Check sheet for the modelled part. Datum: model origin and axes. Units: mm. A direction names the side the tool comes from. Round coordinates to 2 decimals unless told otherwise and drop trailing zeros. Order: outer loops, then holes, each group sorted by start corner. A loop starts at its lowest first (then second) coordinate and runs counter-clockwise, first axis right, second up.
Q1. Depth check by flat-ended pin: P1, Ø12.5, axis at y = 3.5, z = 27, coming from the -X side; P2, Ø8, axis at x = 6, z = 4.5, coming from the +Y side; P3, Ø10, axis at y = 14.5, z = 23, coming from the -X side; P4, Ø5.5, axis at y = -0.5, z = 9.5, coming from the +X side. Enter the tip coordinate at first touch or a pass-through.
Q2. Cross-section at C-C on y = 0. Give the number of separate pieces and of enclosed holes in the cut face, then the cut area to 3 significant figures.
Q3. Cross-section at A-A on y = -16. Record the cut outline in (x, z), then the cut area to 3 significant figures.
Q4. Set-up check for faces 4 (the flat face through (1.5, 0, 27)), 5 (the flat face through (-9, 0, 11)), 6 (the cylindrical face through (-8.4, -6.93, 10.92)), 7 (the cylindrical face through (-3, 0, 28)), 8 (the flat face through (3, -4, 27)): record each of +Z, -Z, +X, -X, +Y, -Y from which the full face is reachable in a straight line by a thin tool's end or side.
Q5. Mould release check, pull along X, two halves, no side actions. Record for faces 1 (the flat face through (0, 7.5, 10)), 2 (the cylindrical face through (8.43, -6.9, 11.08)), 3 (the cylindrical face through (9.84, 9.96, 2.54)): +X half, -X half, draft (parallel to the pull), parting line (faces both ways), or undercut.
Q6. Cross-section at D-D on z = 9. Record the cut outline in (x, y).
Q7. Scan lines: probe 1 along X at (y, z) = (-3.5, 29.5); probe 2 along Z at (x, y) = (15, -11); probe 3 along X at (y, z) = (6.5, 13). Record each from-to range of solid material in increasing order.
from build123d import *

# Parameters (mm, degrees)
SKETCH_R           = 20
PAD_DEPTH          = 5
PAD001_DEPTH       = 7.5
PAD002_DEPTH       = 4
SKETCH003_R        = 2
POCKET_DEPTH       = 24.001
POCKET001_DEPTH    = 27.501
SKETCH005_R        = 2
POCKET002_DEPTH    = 137.001
POLARPATTERN_COUNT = 8
FILLET_R           = 2


with BuildPart() as part:
    # Sketch → Pad (new body)
    with BuildSketch(Plane.XY):
        Circle(SKETCH_R)
    extrude(amount=PAD_DEPTH)

    # Sketch001 → Pad001 (join, symmetric)
    with BuildSketch(Plane.XZ):
        with BuildLine():
            ThreePointArc((9, 17), (0, 26), (-9, 17))
            Line((-9, 5), (-9, 17))
            Line((9, 5), (-9, 5))
            Line((9, 17), (9, 5))
        make_face()
    extrude(amount=PAD001_DEPTH, both=True)

    # Sketch002 → Pad002 (join, symmetric)
    with BuildSketch(Plane.YZ):
        with BuildLine():
            Line((-4, 14), (-4, 30))
            ThreePointArc((4, 30), (0, 34), (-4, 30))
            Line((4, 30), (4, 14))
            Line((4, 14), (-4, 14))
        make_face()
    extrude(amount=PAD002_DEPTH, both=True)

    # Sketch003 (on Face9 of Pad002) → Pocket (cut, through all)
    with BuildSketch(Plane(origin=(-4, 0, 0), x_dir=(0, -1, 0), z_dir=(-1, 0, 0))):
        with Locations((0, 30)):
            Circle(SKETCH003_R)
    extrude(amount=-POCKET_DEPTH, mode=Mode.SUBTRACT)

    # Sketch004 (on Face7 of Pocket) → Pocket001 (cut, through all)
    with BuildSketch(Plane(origin=(0, 7.5, 0), x_dir=(-1, 0, 0), z_dir=(0, 1, 0))):
        with BuildLine():
            ThreePointArc((-1.5, 22.809475), (0, 11), (1.5, 22.809475))
            Line((1.5, 37.2), (1.5, 22.809475))
            Line((-1.5, 37.2), (1.5, 37.2))
            Line((-1.5, 22.809475), (-1.5, 37.2))
        make_face()
    extrude(amount=-POCKET001_DEPTH, mode=Mode.SUBTRACT)

    # Sketch005 (on Face3 of Pocket001) → Pocket002 (cut, through all)
    with BuildSketch(Plane.XY.offset(5)):
        with Locations((16, 0)):
            Circle(SKETCH005_R)
    pocket002 = extrude(amount=-POCKET002_DEPTH, mode=Mode.SUBTRACT)

    # PolarPattern: Pocket002 ×8 about axis
    polarpattern_axis = Axis((0, 0, 5), (0, 0, 1))
    for i in range(1, POLARPATTERN_COUNT):
        add(pocket002.rotate(polarpattern_axis, i * 360 / POLARPATTERN_COUNT), mode=Mode.SUBTRACT)

    # Fillet
    fillet_edges = [part.edges().sort_by_distance(p)[0] for p in [
        (-6.873864, -7.5, 22.809475),
        (6.873864, -7.5, 22.809475),
        (6.873864, 7.5, 22.809475),
        (-6.873864, 7.5, 22.809475),
    ]]
    fillet(fillet_edges, radius=FILLET_R)


solid = part.part
Results found:
1. P1: stops at x = -8.18
1. P2: stops at y = 19.9
1. P3: passes through
1. P4: stops at x = 9
2. separate pieces: 5
2. enclosed holes: 0
2. area: 403 mm2
3. outline: (-12, 0) - (-2, 0) - (-2, 5) - (-12, 5) - close; (2, 0) - (12, 0) - (12, 5) - (2, 5) - close
3. area: 100 mm2
4. face 4: +Z, +Y, -Y
4. face 5: +Z, -X, +Y, -Y
4. face 6: +Z, -X, -Y
4. face 7: +X, -X
4. face 8: +Z, +X, -Y
5. face 1: draft
5. face 2: +X half
5. face 3: undercut
6. outline: (-9, -5.5) arc R2 ccw to (-7, -7.5) - (7, -7.5) arc R2 ccw to (9, -5.5) - (9, 5.5) arc R2 ccw to (7, 7.5) - (-7, 7.5) arc R2 ccw to (-9, 5.5) - close
7. probe 1: x = -4 to -1.5, 1.5 to 4
7. probe 2: z = 0 to 5
7. probe 3: x = -8.73 to -4.47, 4.47 to 8.73
